The drawing under review shows one solid part. Ordinate dimensions are in mm from its lowest x, y, z. Round coordinates to 2 decimals unless told otherwise and drop trailing zeros. Order: outer loops, then holes, each group sorted by start corner. A loop starts at its lowest first (then second) coordinate and runs counter-clockwise, first axis right, second up.
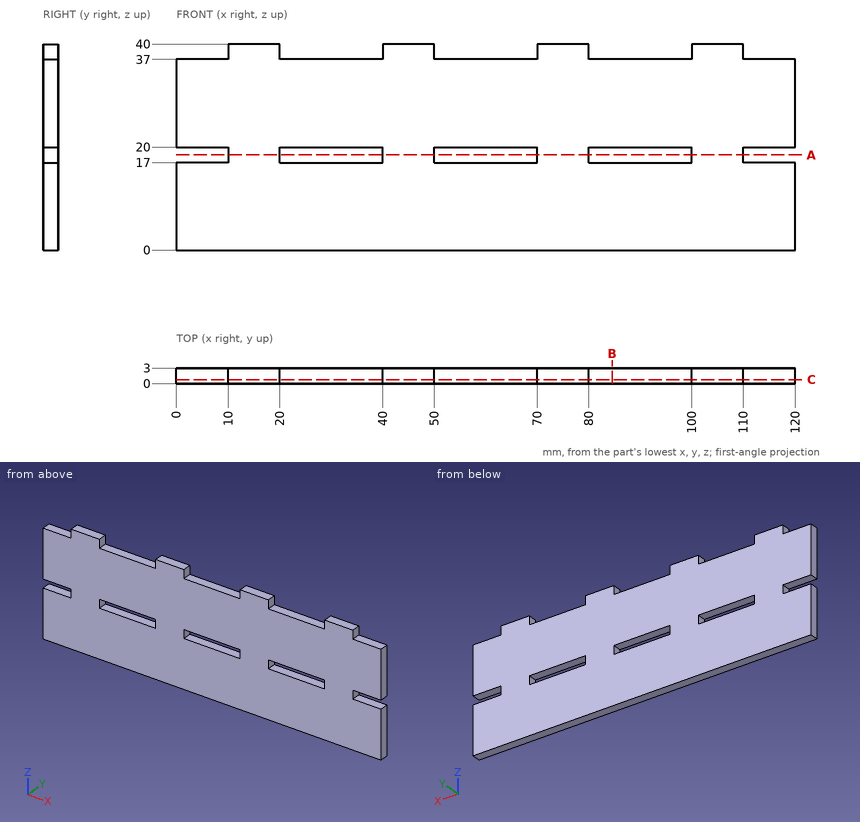
(1) Clearance check with flat-ended pins moving along their axes: P1, Ø1.5, axis at x = 34.5, y = 1, coming from the +Z side; P2, Ø1.5, axis at y = 2, z = 39, coming from the +X side; P3, Ø1.5, axis at y = 1, z = 38, coming from the -X side. State where each tip first meets the part, or that it passes through.
(2) To check wall thickness, follow L1, parallel to Z at x = 67.5, y = 2.45; L2, parallel to X at y = 1.7, z = 18. State the ranges of each line that lie inside material, in increasing order.
(3) We need section C-C (y = 0.8). Count the separate pieces of the cut face and the enclosed holes in it, and give its area (3 significant figures).
(4) We need section A-A (z = 18.5). Give the boundary of the cut face in (x, y), and give its area (3 significant figures).
(5) We need section B-B (x = 84.5). Give the boundary of the cut face in (y, z).
Verdict:
1. P1: stops at z = 37
1. P2: stops at x = 110
1. P3: stops at x = 10
2. L1: z = 0 to 17, 20 to 37
2. L2: x = 10 to 20, 40 to 50, 70 to 80, 100 to 110
3. separate pieces: 1
3. enclosed holes: 3
3. area: 4,320 mm2
4. outline: (10, 0) - (20, 0) - (20, 3) - (10, 3) - close; (40, 0) - (50, 0) - (50, 3) - (40, 3) - close; (70, 0) - (80, 0) - (80, 3) - (70, 3) - close; (100, 0) - (110, 0) - (110, 3) - (100, 3) - close
4. area: 120 mm2
5. outline: (0, 0) - (3, 0) - (3, 17) - (0, 17) - close; (0, 20) - (3, 20) - (3, 37) - (0, 37) - close
